```python
from build123d import *

# Parameters (mm, degrees)
ESBO_O6_W                  = 48
ESBO_O6_H                  = 32
ESBO_O6_W_2                = 17.8
ESBO_O6_H_2                = 13
RESSALTO_EXTRUS_O2_DEPTH   = 3
ESBO_O7_R                  = 1.35
CORTE_EXTRUS_O3_DEPTH      = 30
ESBO_O8_W                  = 48
ESBO_O8_H                  = 3
RESSALTO_EXTRUS_O3_DEPTH   = 13
CORTE_EXTRUS_O4_DEPTH      = 41.902322672
CORTE_EXTRUS_O4_DEPTH_BACK = 41.902322672
ESBO_O10_W                 = 3.1
ESBO_O10_H                 = 3.1
CORTE_EXTRUS_O5_DEPTH      = 41.902322672
CORTE_EXTRUS_O5_DEPTH_BACK = 41.902322672
ESBO_O11_W                 = 30.5
ESBO_O11_H                 = 13
FILETE1_R                  = 6
FILETE2_R                  = 6
FILETE3_R                  = 6


with BuildPart() as part:
    # Esboço6 → Ressalto-extrusão2 (new body)
    with BuildSketch(Plane.XY):
        Rectangle(ESBO_O6_W, ESBO_O6_H)
        Rectangle(ESBO_O6_W_2, ESBO_O6_H_2, mode=Mode.SUBTRACT)
    extrude(amount=RESSALTO_EXTRUS_O2_DEPTH)

    # Esboço7 → Corte-extrusão3 (cut, through all)
    with BuildSketch(Plane.XY.offset(3)):
        with Locations((-19.25, 0)):
            Circle(ESBO_O7_R)
        with Locations(Location((19.25, 0, 0), (0, 0, 180))):
            Circle(ESBO_O7_R)
    extrude(amount=-CORTE_EXTRUS_O3_DEPTH, mode=Mode.SUBTRACT)

    # Esboço8 → Ressalto-extrusão3 (add)
    with BuildSketch(Plane.XY.offset(3)):
        with Locations((0, -14.5)):
            Rectangle(ESBO_O8_W, ESBO_O8_H)
        with Locations((0, 14.5)):
            Rectangle(ESBO_O8_W, ESBO_O8_H)
    extrude(amount=RESSALTO_EXTRUS_O3_DEPTH)

    # Esboço10 → Corte-extrusão4 (cut, two sides: drawn at the far end of the back side and taken through both)
    with BuildSketch(Plane.XZ.offset(-13).offset(-CORTE_EXTRUS_O4_DEPTH_BACK)):
        with Locations((18.5, 9.5)):
            Rectangle(ESBO_O10_W, ESBO_O10_H)
        with Locations((-18.5, 9.5)):
            Rectangle(ESBO_O10_W, ESBO_O10_H)
    extrude(amount=CORTE_EXTRUS_O4_DEPTH + CORTE_EXTRUS_O4_DEPTH_BACK, mode=Mode.SUBTRACT)

    # Esboço11 → Corte-extrusão5 (cut, two sides: drawn at the far end of the back side and taken through both)
    with BuildSketch(Plane.XZ.offset(-13).offset(-CORTE_EXTRUS_O5_DEPTH_BACK)):
        with Locations((0, 9.5)):
            Rectangle(ESBO_O11_W, ESBO_O11_H)
    extrude(amount=CORTE_EXTRUS_O5_DEPTH + CORTE_EXTRUS_O5_DEPTH_BACK, mode=Mode.SUBTRACT)

    # Filete1
    filete1_edges = [part.edges().sort_by_distance(p)[0] for p in [
        (24, -14.5, 16),
    ]]
    fillet(filete1_edges, radius=FILETE1_R)

    # Filete2
    filete2_edges = [part.edges().sort_by_distance(p)[0] for p in [
        (24, 14.5, 16),
    ]]
    fillet(filete2_edges, radius=FILETE2_R)

    # Filete3
    filete3_edges = [part.edges().sort_by_distance(p)[0] for p in [
        (-24, 14.5, 16),
        (-24, -14.5, 16),
    ]]
    fillet(filete3_edges, radius=FILETE3_R)


solid = part.part
```
Geometry check sheet. Reference: the model listing, model coordinates, mm. A direction names the side the tool comes from. Coordinates: 2 decimals unless noted, no trailing zeros. Order: outer loops, then holes, each group sorted by start corner. A loop starts at its lowest first (then second) coordinate and runs counter-clockwise, first axis right, second up.
Q1. Sectioned sample at A-A on z = 8.5. Give the number of separate pieces and of enclosed holes in the cut face, and give its area (3 significant figures).
Reply:
separate pieces: 8
enclosed holes: 0
area: 67.8 mm2
Q2. Sectioned sample at C-C on x = 4. Record the cut outline in (y, z), and give its area (3 significant figures).
Reply:
outline: (-16, 0) - (-6.5, 0) - (-6.5, 3) - (-16, 3) - close; (6.5, 0) - (16, 0) - (16, 3) - (6.5, 3) - close
area: 57.0 mm2
Q3. Thickness scan on probe 1 along Y at (x, z) = (-19.25, 1.85); probe 2 along Z at (x, y) = (-16, 1). Record the ranges inside material, lowest first.
Reply:
probe 1: y = -16 to -1.35, 1.35 to 16
probe 2: z = 0 to 3
Q4. Depth check by flat-ended pin: pin 1 Ø1.5 at (x, y) = (15.5, -3) entering from -Z; pin 2 Ø3 at (x, y) = (-12.5, -4.5) entering from +Z; pin 3 Ø2 at (x, z) = (19, 9) entering from +Y. Enter the tip coordinate at first touch or a pass-through.
Reply:
pin 1: stops at z = 0
pin 2: stops at z = 3
pin 3: passes through
Q5. Tool access check on faces 4 (the face through (-19, 15, 11.05)), 5 (the face through (-0.3, 16, 2.6)). Record the directions out of +Z, -Z, +X, -X, +Y, -Y that give a thin tool (end or side, any length) a straight path to the whole face; none if there is none.
Reply:
face 4: +Y, -Y
face 5: +Z, -Z, +X, -X, +Y
Q6. Sectioned sample at D-D on z = 4.25. Record the cut outline in (x, y), and give its area (3 significant figures).
Reply:
outline: (-24, -16) - (-15.25, -16) - (-15.25, -13) - (-24, -13) - close; (-24, 13) - (-15.25, 13) - (-15.25, 16) - (-24, 16) - close; (15.25, -16) - (24, -16) - (24, -13) - (15.25, -13) - close; (15.25, 13) - (24, 13) - (24, 16) - (15.25, 16) - close
area: 105 mm2
Q7. Draft check along Y on faces 1 (the face through (-0.3, -16, 2.6)), 2 (the face through (-20.05, 15, 9)), 3 (the face through (21, -13, 9)). Enter one of: released by +Y, released by -Y, zero draft, split by the parting line, or undercut.
Reply:
face 1: released by -Y
face 2: zero draft
face 3: undercut
Q8. Sectioned sample at B-B on y = 0. Record the cut outline in (x, z), and give its area (3 significant figures).
Reply:
outline: (-24, 0) - (-20.6, 0) - (-20.6, 3) - (-24, 3) - close; (-17.9, 0) - (-8.9, 0) - (-8.9, 3) - (-17.9, 3) - close; (8.9, 0) - (17.9, 0) - (17.9, 3) - (8.9, 3) - close; (20.6, 0) - (24, 0) - (24, 3) - (20.6, 3) - close
area: 74.4 mm2
